```python
from build123d import *

# Parameters (mm, degrees)
F3_DEPTH = 4
F4_SIZE  = 1
F5_R     = 0.3


with BuildPart() as f1:
    # F0 (on Front) → F1 (revolve)
    with BuildSketch(Plane.XZ):
        Polygon((3.5, 4), (0, 4), (0, -16), (2, -16), (2, 0), (3.5, 0), align=None)
    revolve(axis=Axis((0, 0, -50.553678), (0, 0, -1)))

    # F2 (on face) → F3 (cut)
    with BuildSketch(Plane.XY.offset(4)):
        Polygon((0.866025, 1.5), (-0.866025, 1.5), (-1.732051, 0), (-0.866025, -1.5), (0.866025, -1.5), (1.732051, 0), align=None)
    extrude(amount=-F3_DEPTH, mode=Mode.SUBTRACT)

    # F4
    f4_edges = [f1.edges().sort_by_distance(p)[0] for p in [
        (-2, 0, -16),
    ]]
    chamfer(f4_edges, length=F4_SIZE)

    # F5
    f5_edges = [f1.edges().sort_by_distance(p)[0] for p in [
        (-3.5, 0, 0),
        (-3.5, 0, 4),
    ]]
    fillet(f5_edges, radius=F5_R)


solid = f1.part
```
Design review of the part built by this model. Coordinates are the model's own, in mm. A direction names the side the tool comes from. Coordinates: 2 decimals unless noted, no trailing zeros. Write each loop counter-clockwise with the first axis right and the second up, starting at its lowest first coordinate (ties: lowest second). Pieces come first, ordered by that corner, then holes.
1) Add section C-C (z = -4.5). Write out the cut boundary in (x, y).
2) To check wall thickness, follow L1, parallel to Z at x = -1, y = -3; L2, parallel to X at y = 1, z = -8; L3, parallel to X at y = 1.75, z = -9.75. State the ranges of each line that lie inside material, in increasing order.
3) Add section A-A (z = 0.75). Write out the cut boundary in (x, y), plus the area to 3 significant figures.
4) Insertion check: pin 1 (1.5 mm diameter, centred on y = 0.5, z = -13, fed in from -X); pin 2 (1.5 mm diameter, centred on x = 0.5, y = 0.5, fed in from +Z); pin 3 (1 mm diameter, centred on x = 0.5, y = 2.5, fed in from -Z). Each pin has a flat end and moves straight along its axis. Give the tip position at first contact, or say it passes through.
5) Add section B-B (x = 0). Write out the cut boundary in (y, z), plus the area to 3 significant figures.
6) Machinability: for faces 1 (the cylindrical face through (3.233, 1.341, 2.024)), 2 (the flat face through (1.293, -0.76, 2.028)), 3 (the flat face through (-2, 1, 0)), which of the approach directions +Z, -Z, +X, -X, +Y, -Y give a long, thin tool a straight path to every point of the face, cutting with its end or side? Answer none if there is none.
7) Mouldability with a two-part tool opening along X and no side actions: class faces 4 (the cylindrical face through (0, 2, -7)), 5 (the flat face through (0, 0, 0)), 6 (the flat face through (0, 0, -16)) as +X half, -X half, draft (parallel to the pull), parting line (faces both ways), or undercut.
Check result:
1. outline: circle Ø4 at (0, 0)
2. L1: z = 0 to 4
2. L2: x = -1.73 to 1.73
2. L3: x = -0.97 to 0.97
3. outline: circle Ø7 at (0, 0); hole (-1.73, 0) - (-0.87, -1.5) - (0.87, -1.5) - (1.73, 0) - (0.87, 1.5) - (-0.87, 1.5) - close
3. area: 30.7 mm2
4. pin 1: stops at x = -2
4. pin 2: stops at z = 0
4. pin 3: stops at z = 0
5. outline: (-3.5, 0.3) arc R0.3 ccw to (-3.2, 0) - (-2, 0) - (-2, -15) - (-1, -16) - (1, -16) - (2, -15) - (2, 0) - (3.2, 0) arc R0.3 ccw to (3.5, 0.3) - (3.5, 3.7) arc R0.3 ccw to (3.2, 4) - (1.5, 4) - (1.5, 0) - (-1.5, 0) - (-1.5, 4) - (-3.2, 4) arc R0.3 ccw to (-3.5, 3.7) - close
5. area: 78.9 mm2
6. face 1: +Z, -Z
6. face 2: +Z
6. face 3: -Z
7. face 4: parting line
7. face 5: undercut
7. face 6: draft
